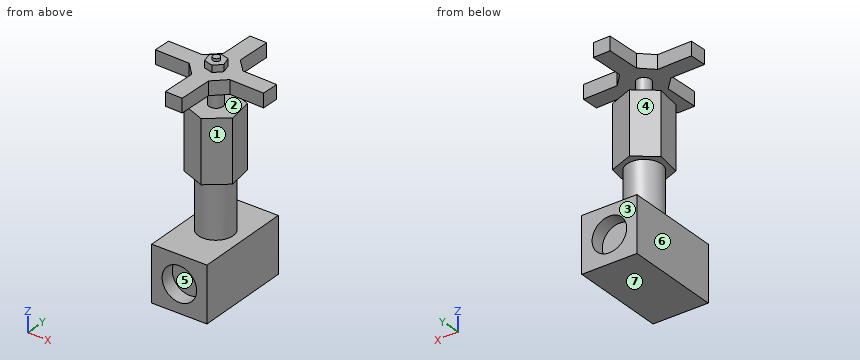
from build123d import *

# Parameters (mm, degrees)
F0_W      = 40
F0_H      = 40
F1_DEPTH  = 70
F2_R      = 12.5
F3_DEPTH  = 10
F4_R      = 12.5
F5_DEPTH  = 10
F6_R      = 12.5
F7_DEPTH  = 40
F9_DEPTH  = 45
F10_R     = 5
F11_DEPTH = 15
F13_DEPTH = 10
F14_W     = 12.4264068712
F14_H     = 10
F15_DEPTH = 25
F16_W     = 12.4264068712
F16_H     = 10
F17_DEPTH = 25
F18_W     = 12.4264068712
F18_H     = 10
F19_DEPTH = 25
F20_W     = 12.4264068712
F20_H     = 10
F21_DEPTH = 25
F23_DEPTH = 5
F24_R     = 2.5
F25_DEPTH = 2


with BuildPart() as f1:
    # F0 (on Front) → F1 (new body)
    with BuildSketch(Plane.XZ):
        Rectangle(F0_W, F0_H)
    extrude(amount=F1_DEPTH)

    # F2 (on Front) → F3 (cut, symmetric)
    with BuildSketch(Plane.XZ):
        Circle(F2_R)
    extrude(amount=F3_DEPTH, both=True, mode=Mode.SUBTRACT)

    # F4 (on face) → F5 (cut, symmetric)
    with BuildSketch(Plane.XZ.offset(70)):
        Circle(F4_R)
    extrude(amount=F5_DEPTH, both=True, mode=Mode.SUBTRACT)

    # F6 (on face) → F7 (join)
    with BuildSketch(Plane.XY.offset(20)):
        with Locations((0, -34.2291915306)):
            Circle(F6_R)
    extrude(amount=F7_DEPTH)

    # F8 (on face) → F9 (join)
    with BuildSketch(Plane.XY.offset(60)):
        Polygon((-2.7817631709, -15.9646048395), (-17.2084776495, -27.5059757583), (-14.4267144786, -45.7705624494), (2.7817631709, -52.4937782216), (17.2084776495, -40.9524073028), (14.4267144786, -22.6878206118), align=None)
    extrude(amount=F9_DEPTH)

    # F10 (on face) → F11 (join)
    with BuildSketch(Plane.XY.offset(105)):
        with Locations((0, -33.963235583)):
            Circle(F10_R)
    extrude(amount=F11_DEPTH)

    # F12 (on face) → F13 (join)
    with BuildSketch(Plane.XY.offset(120)):
        Polygon((15.1713289677, -28.1809631677), (6.6390655572, -19.1468019547), (-5.7822724153, -18.7919066152), (-14.8164336282, -27.3241700258), (-15.1713289677, -39.7455079982), (-6.6390655572, -48.7796692112), (5.7822724153, -49.1345645507), (14.8164336282, -40.6023011401), align=None)
    extrude(amount=F13_DEPTH)

    # F14 (on face) → F15 (join)
    with BuildSketch(Plane(origin=(-1.3979831463, -48.9294144098, 0), x_dir=(0.9995920865, -0.0285597714, 0), z_dir=(-0.0285597714, -0.9995920865, 0))):
        with Locations((0.9699822441, 125)):
            Rectangle(F14_W, F14_H)
    extrude(amount=F15_DEPTH)

    # F16 (on face) → F17 (join)
    with BuildSketch(Plane(origin=(15.9634678733, -0.4560990421, 0), x_dir=(0.0285597714, 0.9995920865, 0), z_dir=(0.9995920865, -0.0285597714, 0))):
        with Locations((-33.9493815218, 125)):
            Rectangle(F16_W, F16_H)
    extrude(amount=F17_DEPTH)

    # F18 (on face) → F19 (join)
    with BuildSketch(Plane(origin=(-14.0242947227, 0.4006940998, 0), x_dir=(-0.0285597714, -0.9995920865, 0), z_dir=(-0.9995920865, 0.0285597714, 0))):
        with Locations((33.9493815218, 125)):
            Rectangle(F18_W, F18_H)
    extrude(amount=F19_DEPTH)

    # F20 (on face) → F21 (join)
    with BuildSketch(Plane(origin=(-0.5411900044, -18.9416518138, 0), x_dir=(-0.9995920865, 0.0285597714, 0), z_dir=(0.0285597714, 0.9995920865, 0))):
        with Locations((-0.9699822441, 125)):
            Rectangle(F20_W, F20_H)
    extrude(amount=F21_DEPTH)

    # F22 (on face) → F23 (join)
    with BuildSketch(Plane.XY.offset(130)):
        Polygon((-1.8446433706, -26.9791675509), (-6.7057435207, -31.9157357243), (-4.8611001501, -38.5938560313), (1.8446433706, -40.335408165), (6.7057435207, -35.3988399916), (4.8611001501, -28.7207196846), align=None)
    extrude(amount=F23_DEPTH)

    # F24 (on face) → F25 (join)
    with BuildSketch(Plane.XY.offset(135)):
        with Locations((0, -33.5882875384)):
            Circle(F24_R)
    extrude(amount=F25_DEPTH)


solid = f1.part
Build history of the part. All positions in model axes, mm. Face numbers are marked on the shaded views. A direction names the side the tool comes from. Give positions to 0.01 mm unless a question says otherwise; leave off trailing zeros. Write each loop counter-clockwise with the first axis right and the second up, starting at its lowest first coordinate (ties: lowest second). Pieces come first, ordered by that corner, then holes. Notation, with made-up numbers: (47, 83) - (73, 83) arc R19 ccw to (73, 106) - close; hole circle Ø2 at (48, 14.25). An arc over 180 degrees is marked (long way). Use one line per item in the form item = value. Start each with the question number.
1. Band-saw the part on A-A on y = -64. Write the cut outline in (x, z).
2. Band-saw the part on B-B on x = -9.5. Write the cut outline in (y, z), plus the area to 3 significant figures.
3. 3-axis set-ups, long thin cutter, end or side, ignore diameter. For the marked faces 1, 2, 3 and 4: which of +Z, -Z, +X, -X, +Y, -Y reach the whole face in a straight line?
4. Band-saw the part on C-C on y = -25. Write the cut outline in (x, z).
5. Drop flat-ended pins along their axis: pin 1 Ø7.5 at (x, z) = (-3, -3.5) entering from +Y; pin 2 Ø12 at (x, z) = (-3.5, -8.5) entering from +Y; pin 3 Ø20 at (x, z) = (0, 0) entering from -Y; pin 4 Ø6 at (y, z) = (-52.5, 50.5) entering from +X. Give the stop position or say it passes through.
6. Two-plate mould, pull along X, no slides. Class the marked faces 5, 6 and 7: released by +X, released by -X, zero draft, split by the parting line, or undercut.
7. Probe line 1 (Z direction, x = 0, y = -63); line 2 (Z direction, x = -2, y = -51.5); line 3 (Z direction, x = 3, y = -38.5). List the from-to ranges inside material, lowest first. Write a range as [from, to].
8. Band-saw the part on D-D on z = 0. Write the cut outline in (x, y), plus the area to 3 significant figures.
Conclusion:
q1.outline = (-20, -20) - (20, -20) - (20, 20) - (-20, 20) - close; (-7.07, 120) - (5.36, 120) - (5.36, 130) - (-7.07, 130) - close; hole circle Ø25 at (0, 0)
q2.outline = (-70, -20) - (0, -20) - (0, -8.12) - (-10, -8.12) - (-10, 8.12) - (0, 8.12) - (0, 20) - (-26.11, 20) - (-26.11, 60) - (-21.34, 60) - (-21.34, 105) - (-47.7, 105) - (-47.7, 60) - (-42.35, 60) - (-42.35, 20) - (-70, 20) - (-70, 8.12) - (-60, 8.12) - (-60, -8.12) - (-70, -8.12) - close; (-45.75, 120) - (-22.3, 120) - (-22.3, 130) - (-45.75, 130) - close
q2.area = 4,550 mm²
q3.face_1 = +X, -Y
q3.face_2 = none
q3.face_3 = -Z, +X, -X, +Y
q3.face_4 = -X, +Y
q4.outline = (-20, -20) - (20, -20) - (20, 20) - (8.43, 20) - (8.43, 60) - (14.78, 60) - (14.78, 105) - (-14.08, 105) - (-14.08, 60) - (-8.43, 60) - (-8.43, 20) - (-20, 20) - close; (-12.36, 120) - (12.17, 120) - (12.17, 130) - (-12.36, 130) - close
q5.pin_1 = -10
q5.pin_2 = 0
q5.pin_3 = -60
q5.pin_4 = through
q6.face_5 = undercut
q6.face_6 = released by -X
q6.face_7 = zero draft
q7.line_1 = [-20, -12.5], [12.5, 20], [120, 130]
q7.line_2 = [-20, 20], [120, 130]
q7.line_3 = [-20, 105], [120, 135]
q8.outline = (-20, -70) - (-12.5, -70) - (-12.5, -60) - (12.5, -60) - (12.5, -70) - (20, -70) - (20, 0) - (12.5, 0) - (12.5, -10) - (-12.5, -10) - (-12.5, 0) - (-20, 0) - close
q8.area = 2,300 mm²
